Can you work these out from the model? Positions are in its coordinate system, mm. Face numbers are marked on the shaded views. A direction names the side the tool comes from. Round coordinates to 2 decimals unless told otherwise and drop trailing zeros. Loops run counter-clockwise (first coordinate to the right, second up) from the corner with the lowest first, then second, coordinate; pieces in that order, holes last.
(1) Thinking about a two-plate mould opening in Z: for the marked faces 5, 6 and 7, which applies, released by +Z, released by -Z, zero draft, split by the parting line, or undercut?
(2) I want a section at B-B on x = 0. Write out the boundary of the cut face in (y, z), plus the area to 3 significant figures.
(3) If I drill on line 1 along X through (y, z) = (6.5, -31.5); line 2 along X through (y, z) = (13, -31); line 3 along X through (y, z) = (8.2, 2.5), over which ranges is the centre line in solid material (lowest first)?
(4) I want a section at A-A on z = 2.5. Write out the boundary of the cut face in (x, y).
(5) Which directions (+Z, -Z, +X, -X, +Y, -Y) give clear straight access to the entire face, cutting with the end or side of a thin tool? Please do the marked faces 1, 2, 3 and 4.
(6) I want a section at D-D on z = -11. Write out the boundary of the cut face in (x, y).
(7) Will these pins go through, and if not, where does the flat tip stop? pin 1 Ø1.2 at (y, z) = (-0.5, -57.5) entering from -X; pin 2 Ø10 at (x, z) = (0.5, -9.5) entering from -Y; pin 3 Ø1.2 at (x, z) = (8.75, -31.5) entering from -Y (3 decimals); pin 4 Ø2.5 at (y, z) = (23.5, -11.5) entering from +X.
(8) I want a section at C-C on y = 18. Write out the boundary of the cut face in (x, z), plus the area to 3 significant figures.
from build123d import *

# Parameters (mm, degrees)
SKETCH1_W             = 22.3
SKETCH1_H             = 37
BOSS_EXTRUDE1_DEPTH   = 20.8
FILLET1_R             = 5
BOSS_EXTRUDE2_DEPTH   = 27.2
SKETCH3_R             = 3.5
BOSS_EXTRUDE3_DEPTH   = 8
CUT_EXTRUDE1_START    = -8
CUT_EXTRUDE1_DEPTH    = 8
SKETCH5_W             = 6
SKETCH5_H             = 3
BOSS_EXTRUDE4_DEPTH   = 5
CUT_EXTRUDE2_REACH    = 69.819
SKETCH7_R             = 1.25
FILLET2_R             = 1
F_2_0MM_DOWEL_HOLE1_D = 2
SKETCH10_W            = 8
SKETCH10_H            = 23.2
BOSS_EXTRUDE5_DEPTH   = 2.5
SKETCH11_R            = 4.5
BOSS_EXTRUDE6_DEPTH   = 0.9


with BuildPart() as part:
    # Sketch1 → Boss-Extrude1 (new body)
    with BuildSketch(Plane(origin=(0, 0, 0), x_dir=(1, 0, 0), z_dir=(0, 1, 0))):
        with Locations((0, 18.5)):
            Rectangle(SKETCH1_W, SKETCH1_H)
    extrude(amount=BOSS_EXTRUDE1_DEPTH)

    # Fillet1
    fillet1_edges = [part.edges().sort_by_distance(p)[0] for p in [
        (11.15, 10.4, 0),
        (-11.15, 10.4, 0),
    ]]
    fillet(fillet1_edges, radius=FILLET1_R)

    # Sketch2 → Boss-Extrude2 (add)
    with BuildSketch(Plane(origin=(0, 0, -37), x_dir=(-1, 0, 0), z_dir=(0, 0, -1))):
        with BuildLine():
            Line((-6.982120022, 0), (6.982120022, 0))
            ThreePointArc((6.982120022, 0), (11, 8.5), (6.982120022, 17))
            Line((6.982120022, 17), (-6.982120022, 17))
            ThreePointArc((-6.982120022, 17), (-11, 8.5), (-6.982120022, 0))
        make_face()
    extrude(amount=BOSS_EXTRUDE2_DEPTH)

    # Sketch3 → Boss-Extrude3 (add)
    with BuildSketch(Plane(origin=(0, 20.8, 0), x_dir=(1, 0, 0), z_dir=(0, 1, 0))):
        with Locations(Location((0, 11, 0), (0, 0, 90))):
            Circle(SKETCH3_R)
    extrude(amount=BOSS_EXTRUDE3_DEPTH)

    # Sketch4 → Cut-Extrude1 (cut)
    with BuildSketch(Plane(origin=(0, 28.8, 0), x_dir=(1, 0, 0), z_dir=(0, 1, 0)).offset(CUT_EXTRUDE1_START)):
        with BuildLine():
            Line((-2.4, 13.547547841), (-2.4, 8.452452159))
            ThreePointArc((-2.4, 8.452452159), (-3.5, 11), (-2.4, 13.547547841))
        make_face()
        with BuildLine():
            Line((2.4, 13.547547841), (2.4, 8.452452159))
            ThreePointArc((2.4, 8.452452159), (3.5, 11), (2.4, 13.547547841))
        make_face()
    extrude(amount=CUT_EXTRUDE1_DEPTH, mode=Mode.SUBTRACT)

    # Sketch5 → Boss-Extrude4 (add)
    with BuildSketch(Plane.XY):
        with Locations((0, 8.5)):
            Rectangle(SKETCH5_W, SKETCH5_H)
    extrude(amount=BOSS_EXTRUDE4_DEPTH)

    # Sketch7 → Cut-Extrude2 (cut, up to next)
    with BuildSketch(Plane(origin=(0, 10, 0), x_dir=(1, 0, 0), z_dir=(0, 1, 0)), mode=Mode.PRIVATE) as cut_extrude2_sk1:
        with Locations(Location((0, -2.5, 0), (0, 0, 270))):
            Circle(SKETCH7_R)
    cut_extrude2_tool1 = extrude(cut_extrude2_sk1.sketch, amount=-CUT_EXTRUDE2_REACH, mode=Mode.PRIVATE) & part.part
    add(cut_extrude2_tool1.solids().sort_by_distance((0, 10, 2.5))[0], mode=Mode.SUBTRACT)

    # Fillet2
    fillet2_edges = [part.edges().sort_by_distance(p)[0] for p in [
        (3, 8.5, 5),
        (-3, 8.5, 5),
    ]]
    fillet(fillet2_edges, radius=FILLET2_R)

    # Ø2.0mm Dowel Hole1 (through all)
    with Locations(Plane(origin=(0, 20.8, 0), x_dir=(1, 0, 0), z_dir=(0, 1, 0))):
        with Locations((-8.75, 31.5), (8.75, 31.5)):
            Hole(F_2_0MM_DOWEL_HOLE1_D / 2)

    # Sketch10 → Boss-Extrude5 (add)
    with BuildSketch(Plane.XZ):
        with Locations((0, -52.6)):
            Rectangle(SKETCH10_W, SKETCH10_H)
    extrude(amount=BOSS_EXTRUDE5_DEPTH)

    # Sketch11 → Boss-Extrude6 (add)
    with BuildSketch(Plane.XZ):
        with Locations(Location((0, -11, 0), (0, 0, 270))):
            Circle(SKETCH11_R)
    extrude(amount=BOSS_EXTRUDE6_DEPTH)


solid = part.part
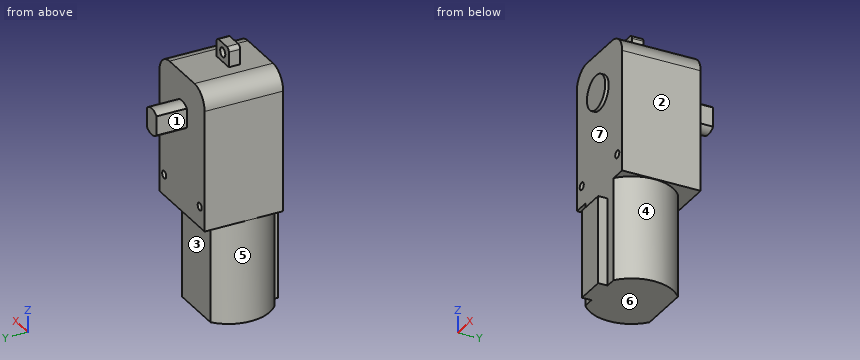
Filled sheet:
1. face 5: zero draft
1. face 6: released by -Z
1. face 7: undercut
2. outline: (-2.5, -64.2) - (17, -64.2) - (17, -37) - (20.8, -37) - (20.8, -14.5) - (28.8, -14.5) - (28.8, -7.5) - (20.8, -7.5) - (20.8, 0) - (10, 0) - (10, 1.25) - (7, 1.25) - (7, 0) - (0, 0) - (0, -6.5) - (-0.9, -6.5) - (-0.9, -15.5) - (0, -15.5) - (0, -41) - (-2.5, -41) - close; (7, 3.75) - (10, 3.75) - (10, 5) - (7, 5) - close
2. area: 1,360 mm2
3. line 1: x = -11.15 to -9.75, -7.75 to 7.75, 9.75 to 11.15
3. line 2: x = -11.15 to -9.62, -7.88 to 7.88, 9.62 to 11.15
3. line 3: x = -3 to -1.25, 1.25 to 3
4. outline: (-3, 7) - (-1.25, 7) - (-1.25, 10) - (-3, 10) - close; (1.25, 7) - (3, 7) - (3, 10) - (1.25, 10) - close
5. face 1: +Z, -Z, -X, +Y
5. face 2: +Z, -Z, +X, +Y, -Y
5. face 3: -Z, +X, -X, +Y
5. face 4: -Z, +X
6. outline: (-11.15, 0) - (-4.5, 0) - (-4.5, -0.9) - (4.5, -0.9) - (4.5, 0) - (11.15, 0) - (11.15, 20.8) - (2.4, 20.8) - (2.4, 28.8) - (-2.4, 28.8) - (-2.4, 20.8) - (-11.15, 20.8) - close
7. pin 1: stops at x = -7.1
7. pin 2: stops at y = -0.9
7. pin 3: passes through
7. pin 4: stops at x = 2.4
8. outline: (-11.15, -37) - (11.15, -37) - (11.15, -5) arc R5 ccw to (6.15, 0) - (-6.15, 0) arc R5 ccw to (-11.15, -5) - close; hole circle Ø2 at (-8.75, -31.5); hole circle Ø2 at (8.75, -31.5)
8. area: 808 mm2
